The model under review builds one solid part; all positions refer to its coordinate system, in mm. Face numbers are marked on the shaded views. A direction names the side the tool comes from. Coordinates: 2 decimals unless noted, no trailing zeros. Order: outer loops, then holes, each group sorted by start corner. A loop starts at its lowest first (then second) coordinate and runs counter-clockwise, first axis right, second up. Notation, with made-up numbers: M 88.5,80.5 L 104.5,80.5 A7 cw 104.5,91.5 Z; hole C 33.5,58.25 d11. An arc over 180 degrees is marked long. Answer in a Markdown table with one row per item.
from build123d import *

# Parameters (mm, degrees)
SKETCH1_W             = 25.4
SKETCH1_H             = 25.4
BOSS_EXTRUDE1_DEPTH   = 6.35
SKETCH2_W             = 25.4
SKETCH2_H             = 31.75
BOSS_EXTRUDE2_DEPTH   = 6.35
FILLET1_R             = 2.54
F_8_CLEARANCE_HOLE1_D = 4.3053
F_8_CLEARANCE_HOLE2_D = 4.3053


with BuildPart() as part:
    # Sketch1 → Boss-Extrude1 (new body)
    with BuildSketch(Plane(origin=(0, 0, 0), x_dir=(1, 0, 0), z_dir=(0, 1, 0))):
        Rectangle(SKETCH1_W, SKETCH1_H)
    extrude(amount=BOSS_EXTRUDE1_DEPTH)

    # Sketch2 → Boss-Extrude2 (add)
    with BuildSketch(Plane(origin=(0, 0, -12.7), x_dir=(-1, 0, 0), z_dir=(0, 0, -1))):
        with Locations((0, 15.875)):
            Rectangle(SKETCH2_W, SKETCH2_H)
    extrude(amount=BOSS_EXTRUDE2_DEPTH)

    # Fillet1
    fillet1_edges = [part.edges().sort_by_distance(p)[0] for p in [
        (0, 31.75, -12.7),
        (-12.7, 31.75, -15.875),
        (12.7, 31.75, -15.875),
        (0, 6.35, 12.7),
        (0, 31.75, -19.05),
        (0, 0, 12.7),
        (12.7, 3.175, 12.7),
        (-12.7, 3.175, 12.7),
        (0, 6.35, -12.7),
    ]]
    fillet(fillet1_edges, radius=FILLET1_R)

    # #8 Clearance Hole1 (through all)
    with Locations(Plane(origin=(0, 6.35, 0), x_dir=(1, 0, 0), z_dir=(0, 1, 0))):
        with Locations((-6.35, 0), (6.35, 0)):
            Hole(F_8_CLEARANCE_HOLE1_D / 2)

    # #8 Clearance Hole2 (through all)
    with Locations(Plane.XY.offset(-12.7)):
        with Locations((6.35, 19.05), (-6.35, 19.05)):
            Hole(F_8_CLEARANCE_HOLE2_D / 2)


solid = part.part
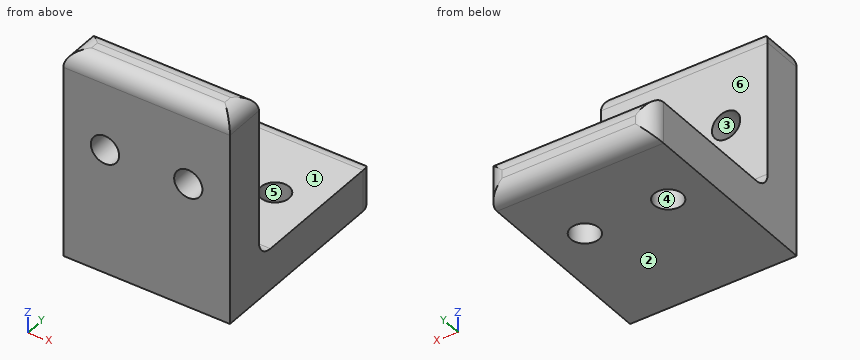
(1) Take a section at B-B (z = 0). Write out the cut boundary in (x, y), then the cut area to 3 significant figures.
Report:
| item | result |
|---|---|
| outline | M -12.7,0 L -8.5,0 L -8.5,6.35 L -12.7,6.35 Z; M -4.2,0 L 4.2,0 L 4.2,6.35 L -4.2,6.35 Z; M 8.5,0 L 12.7,0 L 12.7,6.35 L 8.5,6.35 Z |
| area | 107 mm^2 |
(2) Take a section at A-A (y = 19.05). Write out the cut boundary in (x, z), then the cut area to 3 significant figures.
Report:
| item | result |
|---|---|
| outline | M -12.7,-19.05 L -8.5,-19.05 L -8.5,-12.7 L -12.7,-12.7 Z; M -4.2,-19.05 L 4.2,-19.05 L 4.2,-12.7 L -4.2,-12.7 Z; M 8.5,-19.05 L 12.7,-19.05 L 12.7,-12.7 L 8.5,-12.7 Z |
| area | 107 mm^2 |
(3) Take a section at C-C (x = 6.35). Write out the cut boundary in (y, z).
Report:
| item | result |
|---|---|
| outline | M 0,-19.05 L 16.9,-19.05 L 16.9,-12.7 L 8.89,-12.7 A2.54 cw 6.35,-10.16 L 6.35,-2.15 L 0,-2.15 Z; M 0,2.15 L 6.35,2.15 L 6.35,10.16 A2.54 ccw 3.81,12.7 L 2.54,12.7 A2.54 ccw 0,10.16 Z; M 21.2,-19.05 L 29.21,-19.05 A2.54 ccw 31.75,-16.51 L 31.75,-15.24 A2.54 ccw 29.21,-12.7 L 21.2,-12.7 Z |
(4) To check wall thickness, follow line 1 (X direction, y = 19, z = -15); line 2 (X direction, y = 6, z = -1.5); line 3 (Y direction, x = -6.35, z = -15.5). State the ranges of each line that lie inside material, in increasing order. Write a range as [from, to].
Report:
| item | result |
|---|---|
| line 1 | [-12.7, -8.5], [-4.2, 4.2], [8.5, 12.7] |
| line 2 | [-12.7, -7.89], [-4.81, 4.81], [7.89, 12.7] |
| line 3 | [0, 16.9], [21.2, 31.75] |
(5) The part is to be moulded in two halves that separate along Y. For the marked faces 3, 4, 5 and 6, say which applies: +Y half, -Y half, draft (parallel to the pull), parting line (faces both ways), or undercut.
Report:
| item | result |
|---|---|
| face 3 | draft |
| face 4 | undercut |
| face 5 | undercut |
| face 6 | +Y half |
(6) Insertion check: P1, Ø10, axis at x = -4.5, y = 20, coming from the +Z side; P2, Ø5, axis at x = -6.35, z = 0, coming from the +Y side; P3, Ø10, axis at x = 5, y = 9.5, coming from the +Z side; P4, Ø6, axis at y = 16, z = -7, coming from the -X side. Each pin has a flat end and moves straight along its axis. Give the tip position at first contact, or say it passes through.
Report:
| item | result |
|---|---|
| P1 | z = -12.7 |
| P2 | y = 6.35 |
| P3 | z = 12.6 |
| P4 | through |
(7) Machinability: for the marked faces 1 and 2, which of the approach directions +Z, -Z, +X, -X, +Y, -Y give a long, thin tool a straight path to every point of the face, cutting with its end or side? Answer none if there is none.
Report:
| item | result |
|---|---|
| face 1 | +Z, +X, -X, +Y |
| face 2 | -Z, +X, -X, +Y, -Y |
(8) Take a section at D-D (x = -3.25). Write out the cut boundary in (y, z).
Report:
| item | result |
|---|---|
| outline | M 0,-19.05 L 29.21,-19.05 A2.54 ccw 31.75,-16.51 L 31.75,-15.24 A2.54 ccw 29.21,-12.7 L 8.89,-12.7 A2.54 cw 6.35,-10.16 L 6.35,10.16 A2.54 ccw 3.81,12.7 L 2.54,12.7 A2.54 ccw 0,10.16 Z |
